Can you work these out from the model? Positions are in its coordinate system, mm. Face numbers are marked on the shaded views. A direction names the side the tool comes from. Coordinates: 2 decimals unless noted, no trailing zeros. Loops run counter-clockwise (first coordinate to the right, second up) from the corner with the lowest first, then second, coordinate; pieces in that order, holes last.
```python
from build123d import *

# Parameters (mm, degrees)
F0_W            = 14
F0_H            = 2
F1_DEPTH        = 3
F2_R            = 0.99
F4_DEPTH        = 25
F4_DEPTH_BACK   = 25
F5_R            = 1
F7_DEPTH        = 25
F7_DEPTH_BACK   = 25
F10_D           = 2
F10_DEPTH       = 4
F10_CSINK_D     = 4.1
F10_CSINK_ANGLE = 90
F10_TIP         = 0.600860619


with BuildPart() as f1:
    # F0 (on Top) → F1 (new body)
    with BuildSketch(Plane.XY):
        Polygon((8, 0.4693894553), (12, 5.4693894553), (12, 10.4693894553), (-12, 10.4693894553), (-12, 5.4693894553), (-8, 0.4693894553), align=None)
        with Locations((0, 2.9693894553)):
            Rectangle(F0_W, F0_H, mode=Mode.SUBTRACT)
    extrude(amount=F1_DEPTH)

    # F2
    f2_edges = [f1.edges().sort_by_distance(p)[0] for p in [
        (-7, 3.969389, 1.5),
        (-7, 1.969389, 1.5),
        (7, 3.969389, 1.5),
        (7, 1.969389, 1.5),
    ]]
    fillet(f2_edges, radius=F2_R)

    # F3 (on Right) → F4 (cut, two sides)
    with BuildSketch(Plane.YZ) as f4_sk:
        Polygon((10.9693894553, -0.8042101245), (10.9693894553, 3.1957898755), (8.1685593025, -0.8042101245), align=None)
    extrude(amount=-F4_DEPTH, mode=Mode.SUBTRACT)
    extrude(f4_sk.sketch, amount=F4_DEPTH_BACK, mode=Mode.SUBTRACT)

    # F5
    f5_edges = [f1.edges().sort_by_distance(p)[0] for p in [
        (8, 0.469389, 1.5),
        (-8, 0.469389, 1.5),
    ]]
    fillet(f5_edges, radius=F5_R)

    # F6 (on Right) → F7 (cut, two sides)
    with BuildSketch(Plane.YZ) as f7_sk:
        Polygon((12.1216029626, 3.5), (8.1216029626, 3.5), (12.1216029626, 0.6991698472), align=None)
    extrude(amount=F7_DEPTH, mode=Mode.SUBTRACT)
    extrude(f7_sk.sketch, amount=-F7_DEPTH_BACK, mode=Mode.SUBTRACT)

    # F10
    with Locations(Plane.XY.offset(3)):
        with Locations((-8, 6.5693894553), (8, 6.5693894553)):
            CounterSinkHole(F10_D / 2, F10_CSINK_D / 2, depth=F10_DEPTH, counter_sink_angle=F10_CSINK_ANGLE)
            with Locations((0, 0, -(F10_DEPTH + F10_TIP / 2))):  # 118° drill point
                Cone(0, F10_D / 2, F10_TIP, mode=Mode.SUBTRACT)


solid = f1.part
```
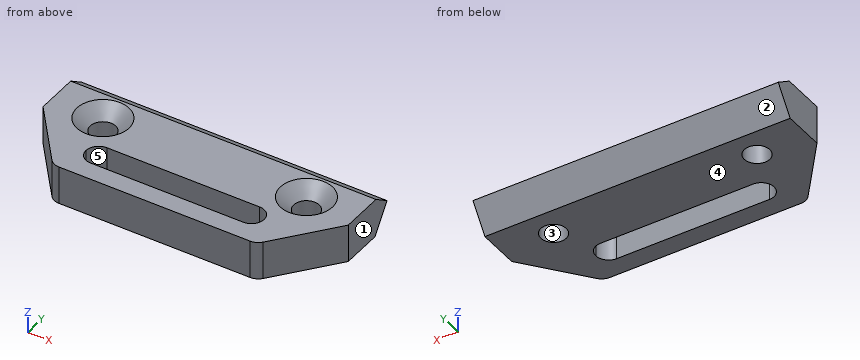
(1) I want a section at C-C on z = 0.7. State how many separate pieces and enclosed holes the cut face has, then the cut area to 3 significant figures.
Check values:
separate pieces: 1
enclosed holes: 3
area: 157 mm2
(2) Which directions (+Z, -Z, +X, -X, +Y, -Y) give clear straight access to the entire face, cutting with the end or side of a thin tool? Please do the marked faces 4 and 5.
Check values:
face 4: -Z, +X, -X, +Y, -Y
face 5: +Z, -Z
(3) If I drill on probe 1 along X at (y, z) = (5.5, 2.85); probe 2 along X at (y, z) = (3, 2.3); probe 3 along X at (y, z) = (3.5, 1.3), over which ranges is the centre line in solid material (lowest first)?
Check values:
probe 1: x = -12 to -9.57, -6.43 to 6.43, 9.57 to 12
probe 2: x = -10.02 to -7, 7 to 10.02
probe 3: x = -10.42 to -6.85, 6.85 to 10.42
(4) If we mould it in two halves opening along X, with no side actions, what happens to the marked faces 1, 2 and 3? For each: released by +X, released by -X, zero draft, split by the parting line, or undercut.
Check values:
face 1: released by +X
face 2: zero draft
face 3: undercut
(5) I want a section at A-A on x = -8. Write out the boundary of the cut face in (y, z).
Check values:
outline: (0.59, 0) - (5.57, 0) - (5.57, 1.95) - (4.52, 3) - (0.59, 3) - close; (7.57, 0) - (8.73, 0) - (10.18, 2.06) - (8.84, 3) - (8.62, 3) - (7.57, 1.95) - close
(6) I want a section at B-B on y = 2.25. Write out the boundary of the cut face in (x, z), then the cut area to 3 significant figures.
Check values:
outline: (-9.42, 0) - (-6.7, 0) - (-6.7, 3) - (-9.42, 3) - close; (6.7, 0) - (9.42, 0) - (9.42, 3) - (6.7, 3) - close
area: 16.3 mm2
(7) I want a section at D-D on x = -5.5. Write out the boundary of the cut face in (y, z), then the cut area to 3 significant figures.
Check values:
outline: (0.47, 0) - (1.97, 0) - (1.97, 3) - (0.47, 3) - close; (3.97, 0) - (8.73, 0) - (10.18, 2.06) - (8.84, 3) - (3.97, 3) - close
area: 21.0 mm2
